Check sheet for the modelled part. Datum: model origin and axes. Units: mm. A direction names the side the tool comes from. Round coordinates to 2 decimals unless told otherwise and drop trailing zeros. Write each loop counter-clockwise with the first axis right and the second up, starting at its lowest first coordinate (ties: lowest second). Pieces come first, ordered by that corner, then holes.
Item 1: Cross-section at D-D on x = 8. Enter the section's corners in (y, z).
Item 2: Release check for a two-part mould opening along X. For faces 1 (the flat face through (35, 0, -20)), 2 (the cylindrical face through (64.297, 23.986, -35.07)), 3 (the flat face through (20, 20, -25)) record: +X half, -X half, draft (parallel to the pull), parting line (faces both ways), or undercut.
Item 3: Material ranges on line 1 (Z direction, x = 55, y = 6.5); line 2 (X direction, y = 27, z = -19); line 3 (Y direction, x = 42.5, z = -38), recorded low to high.
Item 4: Tool access check on faces 4 (the flat face through (52, 20, -30)), 5 (the flat face through (45, 30, -35)), 6 (the flat face through (35, 16, -40)), 7 (the flat face through (30, 30, -28)). Record the directions out of +Z, -Z, +X, -X, +Y, -Y that give a thin tool (end or side, any length) a straight path to the whole face; none if there is none.
Item 5: Cross-section at A-A on z = -13. Enter the section's corners in (x, y) (3 decimals), plus the area to 3 significant figures.
Item 6: Go/stop test with flat-tipped pins: pin 1 Ø6 at (x, z) = (17.5, -28) entering from +Y; pin 2 Ø16 at (x, y) = (50, 23.5) entering from +Z; pin 3 Ø1 at (x, z) = (42, -25.5) entering from -Y; pin 4 Ø4 at (y, z) = (16.5, -11.5) entering from +X. Record where each tip stops, or that it passes through.
Item 7: Cross-section at B-B on y = 21. Enter the section's corners in (x, z), plus the area to 3 significant figures.
Item 8: Cross-section at C-C on x = 55. Enter the section's corners in (y, z).
from build123d import *

# Parameters (mm, degrees)
BOSS_EXTRUDE1_DEPTH            = 40
SKETCH2_W                      = 40
SKETCH2_H                      = 30
BOSS_EXTRUDE2_DEPTH            = 20
BOSS_EXTRUDE3_DEPTH            = 30
CUT_EXTRUDE1_DEPTH             = 30
SKETCH5_W                      = 70
SKETCH5_H                      = 40
BOSS_EXTRUDE4_DEPTH            = 10
SKETCH6_W                      = 20
SKETCH6_H                      = 20
CUT_EXTRUDE2_DEPTH             = 41
F_10_0_10_DIAMETER_HOLE1_D     = 10
F_10_0_10_DIAMETER_HOLE1_DEPTH = 40
FILLET1_R                      = 20


with BuildPart() as part:
    # Sketch1 → Boss-Extrude1 (new body)
    with BuildSketch(Plane(origin=(0, 0, 0), x_dir=(0, -1, 0), z_dir=(-1, 0, 0))):
        Polygon((-10, -4), (-40, -20), (-10, -20), align=None)
    extrude(amount=-BOSS_EXTRUDE1_DEPTH)

    # Sketch2 → Boss-Extrude2 (add)
    with BuildSketch(Plane(origin=(0, 0, -20), x_dir=(-1, 0, 0), z_dir=(0, 0, -1))):
        with Locations((-20, 25)):
            Rectangle(SKETCH2_W, SKETCH2_H)
    extrude(amount=BOSS_EXTRUDE2_DEPTH)

    # Sketch3 → Boss-Extrude3 (add)
    with BuildSketch(Plane(origin=(40, 0, 0), x_dir=(0, 0, -1), z_dir=(1, 0, 0))):
        Polygon((40, 10), (0, 10), (20, 40), (40, 40), align=None)
    extrude(amount=BOSS_EXTRUDE3_DEPTH)

    # Sketch4 → Cut-Extrude1 (cut)
    with BuildSketch(Plane(origin=(70, 0, 0), x_dir=(0, 0, -1), z_dir=(1, 0, 0))):
        Polygon((20, 40), (0, 10), (30, 10), (30, 30), (40, 30), (40, 40), align=None)
    extrude(amount=-CUT_EXTRUDE1_DEPTH, mode=Mode.SUBTRACT)

    # Sketch5 → Boss-Extrude4 (add)
    with BuildSketch(Plane.XZ.offset(-10)):
        with Locations((35, -20)):
            Rectangle(SKETCH5_W, SKETCH5_H)
    extrude(amount=BOSS_EXTRUDE4_DEPTH)

    # Sketch6 → Cut-Extrude2 (cut, through all)
    with BuildSketch(Plane(origin=(0, 0, -40), x_dir=(-1, 0, 0), z_dir=(0, 0, -1))):
        with Locations((-20, 30)):
            Rectangle(SKETCH6_W, SKETCH6_H)
    extrude(amount=-CUT_EXTRUDE2_DEPTH, mode=Mode.SUBTRACT)

    # Ø10.0 (10) Diameter Hole1
    with Locations(Plane(origin=(0, 0, 0), x_dir=(-1, 0, 0), z_dir=(0, -1, 0))):
        with Locations((-55, 15)):
            Hole(F_10_0_10_DIAMETER_HOLE1_D / 2, depth=F_10_0_10_DIAMETER_HOLE1_DEPTH)

    # Fillet1
    fillet1_edges = [part.edges().sort_by_distance(p)[0] for p in [
        (70, 30, -35),
    ]]
    fillet(fillet1_edges, radius=FILLET1_R)


solid = part.part
Response values:
1. outline: (0, -40) - (40, -40) - (40, -20) - (10, -4) - (10, 0) - (0, 0) - close
2. face 1: draft
2. face 2: +X half
2. face 3: undercut
3. line 1: z = -40 to -20, -10 to 0
3. line 2: x = 0 to 10, 30 to 40
3. line 3: y = 0 to 30
4. face 4: +Z, +X, +Y
4. face 5: +Z, -Z, +X, +Y
4. face 6: -Z, +X, -X, +Y, -Y
4. face 7: +Z, -Z, +Y
5. outline: (0, 0) - (50.417, 0) - (50.417, 10) - (40, 10) - (40, 26.875) - (30, 26.875) - (30, 20) - (10, 20) - (10, 26.875) - (0, 26.875) - close; (59.583, 0) - (70, 0) - (70, 10) - (59.583, 10) - close
5. area: 1,150 mm2
6. pin 1: stops at y = 20
6. pin 2: stops at z = -30
6. pin 3: stops at y = 0
6. pin 4: stops at x = 40
7. outline: (0, -40) - (10, -40) - (10, -9.87) - (0, -9.87) - close; (30, -40) - (66.7, -40) - (66.7, -30) - (40, -30) - (40, -9.87) - (30, -9.87) - close
7. area: 870 mm2
8. outline: (0, -40) - (29.36, -40) - (29.36, -30) - (10, -30) - (10, -20) - (0, -20) - close; (0, -10) - (10, -10) - (10, 0) - (0, 0) - close
